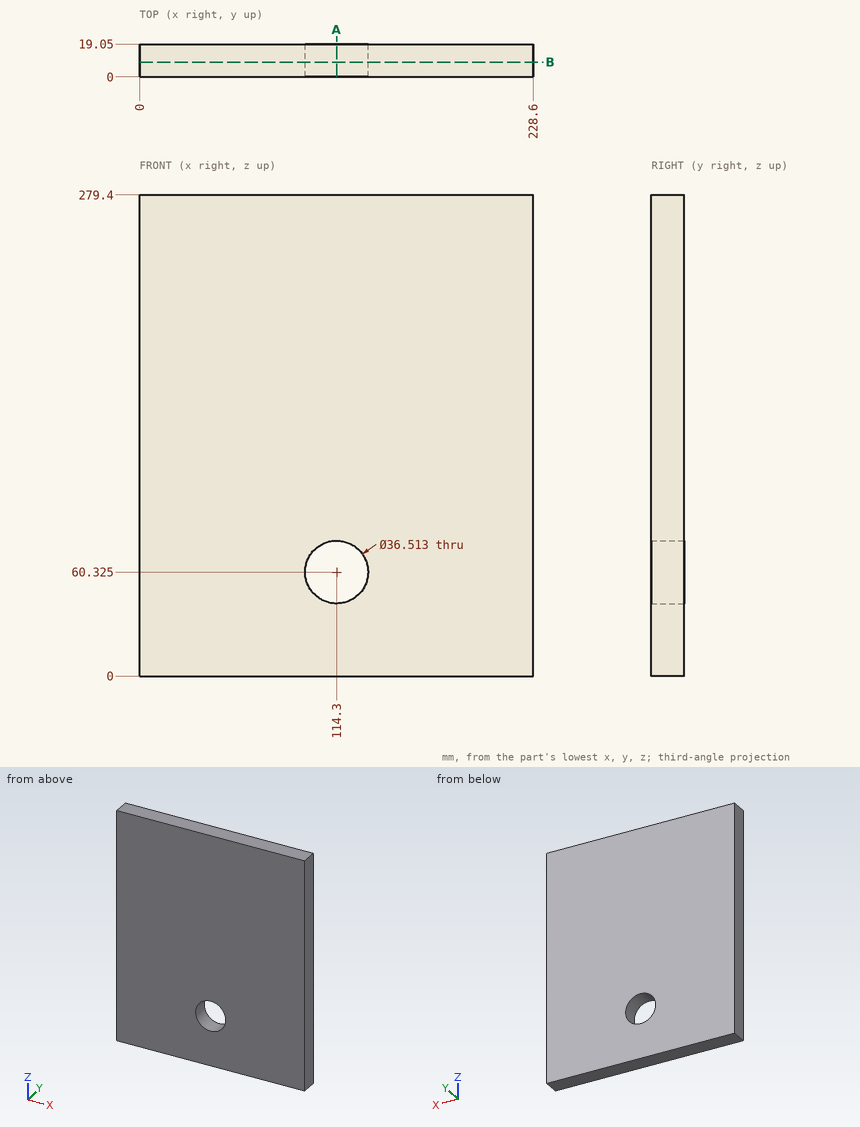
For this review, use the dimensioned drawing (mm, ordinates from the lowest corner) and the shaded views. Coordinates: 2 decimals unless noted, no trailing zeros. Order: outer loops, then holes, each group sorted by start corner. A loop starts at its lowest first (then second) coordinate and runs counter-clockwise, first axis right, second up. Notation, with made-up numbers: (-34, 24.5) - (-30, 24.5) arc R17 cw to (-30, 28.5) - close; hole circle Ø10 at (-5.5, 40). An arc over 180 degrees is marked (long way). Answer in a Markdown table with one row per item.
(1) Wall thickness on line 1 along Z through (x, y) = (114.3, 11.75); line 2 along Z through (x, y) = (128, 18): over which ranges is each line inside the solid? List them lowest first. Write a range as from..to.
Checked values:
| item | result |
|---|---|
| line 1 | 0..42.07, 78.58..279.4 |
| line 2 | 0..48.26, 72.39..279.4 |
(2) Consider section B-B on y = 8.5. State the section outline as (x, z) points (1 decimal), plus the area to 3 significant figures.
Checked values:
| item | result |
|---|---|
| outline | (0, 0) - (228.6, 0) - (228.6, 279.4) - (0, 279.4) - close; hole circle Ø36.5 at (114.3, 60.3) |
| area | 62,800 mm^2 |
(3) Consider section A-A on x = 114.3. State the section outline as (y, z) points.
Checked values:
| item | result |
|---|---|
| outline | (0, 0) - (19.05, 0) - (19.05, 42.07) - (0, 42.07) - close; (0, 78.58) - (19.05, 78.58) - (19.05, 279.4) - (0, 279.4) - close |
(4) Clearance check with a flat-ended pin moving along its axis: pin 1 (2 mm diameter, centred on x = 85.5, y = 13, fed in from -Z). State where the tip first meets the part, or that it passes through.
Checked values:
| item | result |
|---|---|
| pin 1 | z = 0 |
